Can you work these out from the drawing? Everything is in mm from the part's minimum corner. A direction names the side the tool comes from. Give positions to 0.01 mm unless a question says otherwise; leave off trailing zeros. Loops run counter-clockwise (first coordinate to the right, second up) from the corner with the lowest first, then second, coordinate; pieces in that order, holes last. Notation, with made-up numbers: (54.25, 61) - (86.25, 61) arc R21 cw to (86.25, 72) - close; hole circle Ø11 at (39.5, -10). An arc over 180 degrees is marked (long way). Write each question's results on one line, items separated by ' | '. Start each with the question number.
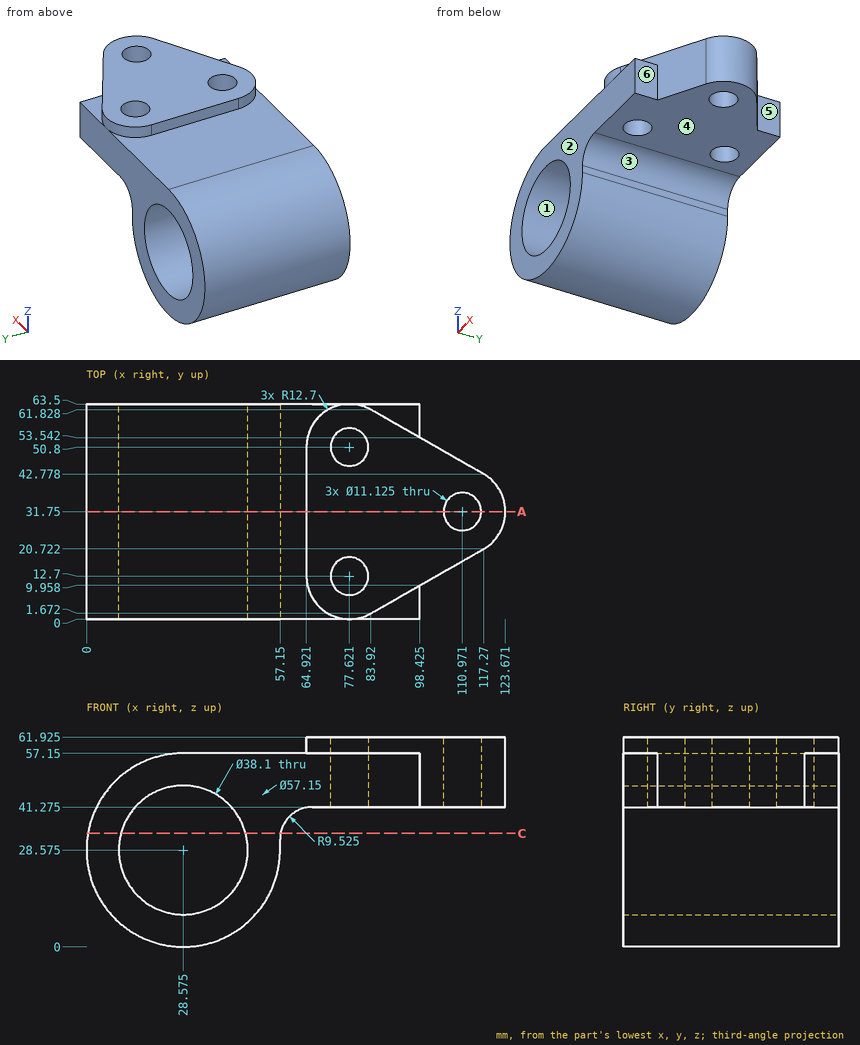
Q1. I want a section at C-C, the plane z = 33.5. List the corners of the cut face in (x, y) for me.
Q2. Which directions (+Z, -Z, +X, -X, +Y, -Y) give clear straight access to the entire face, cutting with the end or side of a thin tool? Please do the marked faces 4, 5 and 6.
Q3. If we mould it in two halves opening along X, with no side actions, what happens to the marked faces 1, 2 and 3? For each: +X half, -X half, draft (parallel to the pull), parting line (faces both ways), or undercut.
Q4. I'm going to push flat-ended pins straight in: pin 1 Ø10 at (y, z) = (47, 41.5) entering from -X; pin 2 Ø10 at (y, z) = (50, 47) entering from -X; pin 3 Ø6 at (y, z) = (18, 50.5) entering from -X (1 decimal); pin 4 Ø14.5 at (x, y) = (110.97, 31.75) entering from +Z (1 decimal). Where does each tip first touch, or does it pass through?
Q5. I want a section at A-A, the plane y = 31.75. State how many separate pieces and enclosed holes the cut face has, then the cut area to 3 significant figures.
Q6. I need wall thicknesses on L1, parallel to Y at x = 81.5, z = 49 (1 decimal); L2, parallel to X at y = 32, z = 43.5 (1 decimal); L3, parallel to Z at x = 100, y = 37 (1 decimal). Which ranges of each line are inside material? Lowest first, please. Write a range as from..to.
Conclusion:
1) outline: (0.43, 0) - (10.17, 0) - (10.17, 63.5) - (0.43, 63.5) - close; (46.98, 0) - (57.31, 0) - (57.31, 63.5) - (46.98, 63.5) - close
2) face 4: -Z, +X, +Y, -Y | face 5: +Z, -Z, +X, +Y | face 6: +Z, -Z, +X, -Y
3) face 1: undercut | face 2: draft | face 3: +X half
4) pin 1: x = 1.12 | pin 2: x = 3.35 | pin 3: x = 7.2 | pin 4: z = 61.9
5) separate pieces: 2 | enclosed holes: 1 | area: 2,730 mm^2
6) L1: 0..8.7, 16.7..46.8, 54.8..63.5 | L2: 4.2..16.7, 40.4..105.4, 116.5..123.7 | L3: 41.3..61.9
